```python
from build123d import *

# Parameters (mm, degrees)
SKETCH1_W           = 177.8
SKETCH1_H           = 25.4
BOSS_EXTRUDE1_DEPTH = 6.35
SKETCH2_R           = 3.175
SKETCH2_R_2         = 6.35
CUT_EXTRUDE1_DEPTH  = 91.02678768
SKETCH3_R           = 9.525
CUT_EXTRUDE2_DEPTH  = 3.571875
SKETCH4_R           = 3.175
CUT_EXTRUDE3_DEPTH  = 91.02678768
CUT_EXTRUDE4_DEPTH  = 91.02678768
FILLET1_R           = 1.27


with BuildPart() as part:
    # Sketch1 → Boss-Extrude1 (new body)
    with BuildSketch(Plane(origin=(0, 0, 0), x_dir=(1, 0, 0), z_dir=(0, 1, 0))):
        Rectangle(SKETCH1_W, SKETCH1_H)
    extrude(amount=BOSS_EXTRUDE1_DEPTH)

    # Sketch2 → Cut-Extrude1 (cut, through all)
    with BuildSketch(Plane(origin=(0, 6.35, 0), x_dir=(1, 0, 0), z_dir=(0, 1, 0))):
        with Locations(Location((-76.2, 0, 0), (0, 0, 270))):
            Circle(SKETCH2_R)
        with Locations(Location((76.2, 0, 0), (0, 0, 270))):
            Circle(SKETCH2_R_2)
        with Locations(Location((-50.8, 0, 0), (0, 0, 270))):
            Circle(SKETCH2_R)
    extrude(amount=-CUT_EXTRUDE1_DEPTH, mode=Mode.SUBTRACT)

    # Sketch3 → Cut-Extrude2 (cut)
    with BuildSketch(Plane(origin=(0, 6.35, 0), x_dir=(1, 0, 0), z_dir=(0, 1, 0))):
        with Locations(Location((76.2, 0, 0), (0, 0, 270))):
            Circle(SKETCH3_R)
    extrude(amount=-CUT_EXTRUDE2_DEPTH, mode=Mode.SUBTRACT)

    # Sketch4 → Cut-Extrude3 (cut, through all)
    with BuildSketch(Plane(origin=(0, 6.35, 0), x_dir=(1, 0, 0), z_dir=(0, 1, 0))):
        with Locations(Location((50.8, 0, 0), (0, 0, 270))):
            Circle(SKETCH4_R)
        with Locations(Location((31.75, 0, 0), (0, 0, 270))):
            Circle(SKETCH4_R)
    extrude(amount=-CUT_EXTRUDE3_DEPTH, mode=Mode.SUBTRACT)

    # Sketch5 → Cut-Extrude4 (cut, through all)
    with BuildSketch(Plane(origin=(0, 6.35, 0), x_dir=(1, 0, 0), z_dir=(0, 1, 0))):
        with BuildLine():
            Line((88.9, 12.7), (76.2, 12.7))
            ThreePointArc((76.2, 12.7), (85.180256121, 8.980256121), (88.9, 0))
            Line((88.9, 0), (88.9, 12.7))
        make_face()
        with BuildLine():
            ThreePointArc((88.9, 0), (85.180256121, -8.980256121), (76.2, -12.7))
            Line((76.2, -12.7), (88.9, -12.7))
            Line((88.9, -12.7), (88.9, 0))
        make_face()
        with BuildLine():
            ThreePointArc((-88.9, 0), (-85.180256121, 8.980256121), (-76.2, 12.7))
            Line((-76.2, 12.7), (-88.9, 12.7))
            Line((-88.9, 12.7), (-88.9, 0))
        make_face()
        with BuildLine():
            Line((-88.9, -12.7), (-76.2, -12.7))
            ThreePointArc((-76.2, -12.7), (-85.180256121, -8.980256121), (-88.9, 0))
            Line((-88.9, 0), (-88.9, -12.7))
        make_face()
    extrude(amount=-CUT_EXTRUDE4_DEPTH, mode=Mode.SUBTRACT)

    # Fillet1
    fillet1_edges = [part.edges().sort_by_distance(p)[0] for p in [
        (0, 0, -12.7),
        (0, 0, 12.7),
        (0, 6.35, 12.7),
        (0, 6.35, -12.7),
        (88.9, 6.35, 0),
        (88.9, 0, 0),
        (-88.9, 6.35, 0),
        (-88.9, 0, 0),
    ]]
    fillet(fillet1_edges, radius=FILLET1_R)

    # Sketch6 → Cut-Revolve2 (revolve, cut)
    with BuildSketch(Plane.ZY.offset(-76.2)):
        Polygon((-8.06821119, 0), (-6.35, 0), (-6.35, 2.778125), (-6.831310248, 2.778125), align=None)
    revolve(axis=Axis((76.2, 0, 0), (0, 1, 0)), mode=Mode.SUBTRACT)


solid = part.part
```
Input: part model. Units: mm. Frame: model coordinates. A direction names the side the tool comes from. Coordinates: 2 decimals unless noted, no trailing zeros. Write each loop counter-clockwise with the first axis right and the second up, starting at its lowest first coordinate (ties: lowest second). Pieces come first, ordered by that corner, then holes.
1) Pin query (flat end, axial travel): pin 1 Ø5.5 at (x, z) = (78.5, 4.5) entering from +Y; pin 2 Ø4 at (x, z) = (62, 4) entering from -Y; pin 3 Ø3 at (y, z) = (4, 5) entering from +X. Return the tip coordinate at first contact, or that it passes through.
2) Material intervals for line 1 along X through (y, z) = (6, 2); line 2 along Y through (x, z) = (50, -11.5); line 3 along X through (y, z) = (3, 7.5), sorted ascending.
3) Section A-A on x = 50.8. Output: boundary loops of the cut face in (y, z) (3 decimals), and give its area (3 significant figures).
4) Mould query, pull axis X, two halves, no side actions, for faces 3 (the flat face through (-1, 3, 12.7)), 4 (the cylindrical face through (67.75, 4.59, 4.4)). Classes: pulls with the +X half, pulls with the -X half, needs draft (parallel to the pull), parting line crosses it, or undercut.
5) Set-up query: faces 1 (the flat face through (-1, 6.35, 0)), 2 (the flat face through (83, 2.778, -2)). Return all of +Z, -Z, +X, -X, +Y, -Y with unobstructed straight access to the full face (end or side cutting, diameter ignored); none if empty.
Check result:
1. pin 1: stops at y = 2.78
1. pin 2: stops at y = 0
1. pin 3: stops at x = 88.41
2. line 1: x = -88.34 to -78.67, -73.73 to -53.27, -48.33 to 29.28, 34.22 to 48.33, 53.27 to 66.89, 85.51 to 88.34
2. line 2: y = 0 to 6.35
2. line 3: x = -86.45 to 70.33, 82.07 to 86.45
3. outline: (0, -11.43) arc R1.27 ccw to (1.27, -12.7) - (5.08, -12.7) arc R1.27 ccw to (6.35, -11.43) - (6.35, -3.175) - (0, -3.175) - close; (0, 3.175) - (6.35, 3.175) - (6.35, 11.43) arc R1.27 ccw to (5.08, 12.7) - (1.27, 12.7) arc R1.27 ccw to (0, 11.43) - close
3. area: 120 mm2
4. face 3: needs draft
4. face 4: undercut
5. face 1: +Z, -Z, +X, -X, +Y
5. face 2: +Y
